from build123d import *

# Parameters (mm, degrees)
BOSS_EXTRUDE1_DEPTH       = 6
SKETCH4_R                 = 2.5
CUT_EXTRUDE1_DEPTH        = 6
SKETCH5_R                 = 2.5
CUT_EXTRUDE2_DEPTH        = 6
F_3_CLEARANCE_HOLE1_D     = 2.794
F_3_CLEARANCE_HOLE1_DEPTH = 6
F_3_CLEARANCE_HOLE1_TIP   = 0.839402285
F_3_CLEARANCE_HOLE2_D     = 2.794
F_3_CLEARANCE_HOLE2_DEPTH = 6
F_3_CLEARANCE_HOLE2_TIP   = 0.839402285
CUT_EXTRUDE3_START        = -2
SKETCH11_R                = 2.5
CUT_EXTRUDE3_DEPTH        = 2
CUT_EXTRUDE4_START        = -2
SKETCH12_R                = 2.5
CUT_EXTRUDE4_DEPTH        = 2


with BuildPart() as part:
    # Sketch3 → Boss-Extrude1 (new, symmetric)
    with BuildSketch(Plane(origin=(0, 0, 0), x_dir=(0, 0, -1), z_dir=(1, 0, 0))):
        with BuildLine():
            Line((-16.237976321, -5.625), (-3.247595264, 16.875))
            ThreePointArc((-3.247595264, 16.875), (0, 18.75), (3.247595264, 16.875))
            Line((3.247595264, 16.875), (16.237976321, -5.625))
            ThreePointArc((16.237976321, -5.625), (16.237976321, -9.375), (12.990381057, -11.25))
            Line((12.990381057, -11.25), (-12.990381057, -11.25))
            ThreePointArc((-12.990381057, -11.25), (-16.237976321, -9.375), (-16.237976321, -5.625))
        make_face()
    extrude(amount=BOSS_EXTRUDE1_DEPTH, both=True)

    # Sketch4 → Cut-Extrude1 (cut)
    with BuildSketch(Plane(origin=(6, 0, 0), x_dir=(0, 0, -1), z_dir=(1, 0, 0))):
        with Locations((0, 15)):
            Circle(SKETCH4_R)
        with Locations((-12.990381057, -7.5)):
            Circle(SKETCH4_R)
        with Locations((12.990381057, -7.5)):
            Circle(SKETCH4_R)
    extrude(amount=-CUT_EXTRUDE1_DEPTH, mode=Mode.SUBTRACT)

    # Sketch5 → Cut-Extrude2 (cut)
    with BuildSketch(Plane.ZY.offset(6)):
        Circle(SKETCH5_R)
    extrude(amount=-CUT_EXTRUDE2_DEPTH, mode=Mode.SUBTRACT)

    # #3 Clearance Hole1
    with Locations(Plane(origin=(0, 0, 0), x_dir=(0, 0, -1), z_dir=(1, 0, 0))):
        with Locations((12.990381057, -7.5), (0, 15), (-12.990381057, -7.5)):
            Hole(F_3_CLEARANCE_HOLE1_D / 2, depth=F_3_CLEARANCE_HOLE1_DEPTH)
            with Locations((0, 0, -(F_3_CLEARANCE_HOLE1_DEPTH + F_3_CLEARANCE_HOLE1_TIP / 2))):  # 118° drill point
                Cone(0, F_3_CLEARANCE_HOLE1_D / 2, F_3_CLEARANCE_HOLE1_TIP, mode=Mode.SUBTRACT)

    # #3 Clearance Hole2
    with Locations(Plane.ZY):
        with Locations((0, 0)):
            Hole(F_3_CLEARANCE_HOLE2_D / 2, depth=F_3_CLEARANCE_HOLE2_DEPTH)
            with Locations((0, 0, -(F_3_CLEARANCE_HOLE2_DEPTH + F_3_CLEARANCE_HOLE2_TIP / 2))):  # 118° drill point
                Cone(0, F_3_CLEARANCE_HOLE2_D / 2, F_3_CLEARANCE_HOLE2_TIP, mode=Mode.SUBTRACT)

    # Sketch11 → Cut-Extrude3 (cut)
    with BuildSketch(Plane.ZY.offset(6).offset(CUT_EXTRUDE3_START)):
        with Locations(Location((0, 15, 0), (0, 0, 180))):
            Circle(SKETCH11_R)
        with Locations(Location((-12.990381057, -7.5, 0), (0, 0, 180))):
            Circle(SKETCH11_R)
        with Locations(Location((12.990381057, -7.5, 0), (0, 0, 180))):
            Circle(SKETCH11_R)
    extrude(amount=CUT_EXTRUDE3_DEPTH, mode=Mode.SUBTRACT)

    # Sketch12 → Cut-Extrude4 (cut)
    with BuildSketch(Plane(origin=(6, 0, 0), x_dir=(0, 0, -1), z_dir=(1, 0, 0)).offset(CUT_EXTRUDE4_START)):
        with Locations(Location((0, 0, 0), (0, 0, 180))):
            Circle(SKETCH12_R)
    extrude(amount=CUT_EXTRUDE4_DEPTH, mode=Mode.SUBTRACT)


solid = part.part
Could you check a few things on this model? Use its own coordinates, in mm. A direction names the side the tool comes from. Give positions to 0.01 mm unless a question says otherwise; leave off trailing zeros. Order: outer loops, then holes, each group sorted by start corner. A loop starts at its lowest first (then second) coordinate and runs counter-clockwise, first axis right, second up.
1. For faces 1 (the cylindrical face through (0.084, -9.327, -16.265)), 2 (the flat face through (0, -9, -14)), 3 (the flat face through (0, -1.1, 1.1)), which set-ups out of +Z, -Z, +X, -X, +Y, -Y let a thin tool reach every point of the face, with its end or its side?
2. We'd pull the mould along Y, two halves only. Please class faces 4 (the flat face through (6, -3, 0)), 5 (the cylindrical face through (0.08, 18.75, 0.05)), 6 (the cylindrical face through (3.04, -9.94, -12.45)), 7 (the cylindrical face through (3.04, 12.56, 0.54)): pulls with the +Y half, pulls with the -Y half, needs draft (parallel to the pull), parting line crosses it, or undercut.
3. Suppose I cut it at C-C (y = 15). List the corners of the cut face in (x, z) for me.
4. Suppose I cut it at D-D (z = -12.5). List the corners of the cut face in (x, y) for me, plus the area to 3 significant figures.
5. I need wall thicknesses on L1, parallel to Z at x = 4.5, y = -9.5; L2, parallel to Y at x = 1.5, z = 1; L3, parallel to Z at x = 5, y = 13. Which ranges of each line are inside material? Lowest first, please.
6. Suppose I cut it at A-A (x = -2.75). List the corners of the cut face in (y, z) for me (3 decimals).
7. Will these pins go through, and if not, where does the flat tip stop? P1, Ø2, axis at x = -1, y = 0, coming from the -Z side; P2, Ø3, axis at y = 15, z = 0, coming from the +X side; P3, Ø1.5, axis at y = -6.5, z = 13, coming from the -X side; P4, Ø2, axis at y = -7.5, z = 12.99, coming from the -X side.
8. Suppose I cut it at B-B (y = -7.5). List the corners of the cut face in (x, z) for me.
Solved:
1. face 1: -Z, +X, -X
1. face 2: +X
1. face 3: -X
2. face 4: needs draft
2. face 5: pulls with the +Y half
2. face 6: undercut
2. face 7: undercut
3. outline: (-6, -4.33) - (6, -4.33) - (6, -2.5) - (0, -2.5) - (0, -1.4) - (-4, -1.4) - (-4, -2.5) - (-6, -2.5) - close; (-6, 2.5) - (-4, 2.5) - (-4, 1.4) - (0, 1.4) - (0, 2.5) - (6, 2.5) - (6, 4.33) - (-6, 4.33) - close
4. outline: (-6, -11.25) - (6, -11.25) - (6, -9.95) - (0, -9.95) - (0, -8.81) - (-4, -8.81) - (-4, -9.95) - (-6, -9.95) - close; (-6, -5.05) - (-4, -5.05) - (-4, -6.19) - (0, -6.19) - (0, -5.05) - (6, -5.05) - (6, 0.85) - (-6, 0.85) - close
4. area: 95.5 mm2
5. L1: z = -16.16 to -14.49, -11.49 to 11.49, 14.49 to 16.16
5. L2: y = -11.25 to -0.98, 0.98 to 12.71, 17.29 to 18.61
5. L3: z = -5.48 to -1.5, 1.5 to 5.48
6. outline: (-11.25, -12.99) arc R3.75 ccw to (-5.625, -16.238) - (16.875, -3.248) arc R3.75 ccw to (16.875, 3.248) - (-5.625, 16.238) arc R3.75 ccw to (-11.25, 12.99) - close; hole circle Ø2.794 at (-7.5, -12.99); hole circle Ø2.794 at (-7.5, 12.99); hole circle Ø5 at (0, 0); hole circle Ø2.794 at (15, 0)
7. P1: stops at z = -13.57
7. P2: stops at x = 0
7. P3: stops at x = -4
7. P4: passes through
8. outline: (-6, -16.74) - (6, -16.74) - (6, -15.49) - (0, -15.49) - (0, -14.39) - (-4, -14.39) - (-4, -15.49) - (-6, -15.49) - close; (-6, -10.49) - (-4, -10.49) - (-4, -11.59) - (0, -11.59) - (0, -10.49) - (6, -10.49) - (6, 10.49) - (0, 10.49) - (0, 11.59) - (-4, 11.59) - (-4, 10.49) - (-6, 10.49) - close; (-6, 15.49) - (-4, 15.49) - (-4, 14.39) - (0, 14.39) - (0, 15.49) - (6, 15.49) - (6, 16.74) - (-6, 16.74) - close
